from build123d import *

# Parameters (mm, degrees)
CHAMFER1_SIZE  = 0.25
FILLET1_R      = 1
SKETCH2_R      = 4
EXTRUDE1_DEPTH = 13
SKETCH3_R      = 3
EXTRUDE2_DEPTH = 8
SKETCH4_R      = 2.5
EXTRUDE3_DEPTH = 3
CHAMFER2_SIZE  = 1
CHAMFER3_SIZE2 = 0.5
CHAMFER3_SIZE  = 1
HOLEWZD1_D     = 2.5
HOLEWZD1_DEPTH = 5.5
HOLEWZD1_TIP   = 0.751075774


with BuildPart() as part:
    # Sketch1 → Revolve1 (revolve)
    with BuildSketch(Plane.XY, mode=Mode.PRIVATE) as revolve1_sk:
        Polygon((0, 0), (31, 0), (31, 12), (13.2, 12), (13.2, 10.7), (12, 10.7), (12, 12), (11, 12), (11, 6), (10, 6), (10, 2), (0, 2), align=None)
    revolve(revolve1_sk.sketch.rotate(Axis((0, 0, 0), (-1, 0, 0)), 90), axis=Axis((0, 0, 0), (-1, 0, 0)))

    # Chamfer1
    chamfer1_edges = [part.edges().sort_by_distance(p)[0] for p in [
        (0, 0, 2),
    ]]
    chamfer(chamfer1_edges, length=CHAMFER1_SIZE)

    # Fillet1
    fillet1_edges = [part.edges().sort_by_distance(p)[0] for p in [
        (31, 0, 12),
    ]]
    fillet(fillet1_edges, radius=FILLET1_R)

    # Sketch2 → Extrude1 (add)
    with BuildSketch(Plane(origin=(0, 0, 0), x_dir=(1, 0, 0), z_dir=(0, 1, 0))):
        with Locations(Location((25, 0, 0), (0, 0, 270))):
            Circle(SKETCH2_R)
    extrude(amount=-EXTRUDE1_DEPTH)

    # Sketch3 → Extrude2 (add)
    with BuildSketch(Plane.XZ.offset(13)):
        with Locations(Location((25, 0, 0), (0, 0, 90))):
            Circle(SKETCH3_R)
    extrude(amount=EXTRUDE2_DEPTH)

    # Sketch4 → Extrude3 (add)
    with BuildSketch(Plane.XZ.offset(21)):
        with Locations(Location((25, 0, 0), (0, 0, 270))):
            Circle(SKETCH4_R)
    extrude(amount=EXTRUDE3_DEPTH)

    # Chamfer2
    chamfer2_edges = [part.edges().sort_by_distance(p)[0] for p in [
        (25, -13, -4),
    ]]
    chamfer(chamfer2_edges, length=CHAMFER2_SIZE - 0.0001)  # a hair under: the kernel refuses the full size

    # Chamfer3
    chamfer3_edges = [part.edges().sort_by_distance(p)[0] for p in [
        (25, -21, -3),
    ]]
    chamfer3_side = [part.faces().sort_by_distance(p)[0] for p in [
        (25, -20.99, -3),
    ]]
    chamfer(chamfer3_edges, length=CHAMFER3_SIZE - 0.0001, length2=CHAMFER3_SIZE2 - 0.0001, reference=chamfer3_side[0])  # a hair under: the kernel refuses the full size

    # HoleWzd1
    with Locations(Plane.ZY.offset(-11)):
        with Locations((0, 9), (7.794228634, -4.5), (-7.794228634, -4.5)):
            Hole(HOLEWZD1_D / 2, depth=HOLEWZD1_DEPTH)
            with Locations((0, 0, -(HOLEWZD1_DEPTH + HOLEWZD1_TIP / 2))):  # 118° drill point
                Cone(0, HOLEWZD1_D / 2, HOLEWZD1_TIP, mode=Mode.SUBTRACT)


solid = part.part
Could you check a few things on this model? Use its own coordinates, in mm. A direction names the side the tool comes from. Round coordinates to 2 decimals unless told otherwise and drop trailing zeros. Loops run counter-clockwise (first coordinate to the right, second up) from the corner with the lowest first, then second, coordinate; pieces in that order, holes last. Notation, with made-up numbers: (-12, -8) - (21, -8) arc R18 cw to (21, 17) - close; hole circle Ø6 at (80.5, -20.75). An arc over 180 degrees is marked (long way). Write item = value, one per line.
1) Imagine slicing it at D-D (y = -18). Please give me the cut outline in (x, z), and give its area (3 significant figures).
Computed:
outline = circle Ø6 at (25, 0)
area = 28.3 mm2
2) On a 3-axis mill with a long thin cutter (end or side, diameter ignored), from which of +Z, -Z, +X, -X, +Y, -Y can I reach the whole of each face in a straight line? I mean faces 1 (the flat face through (0, 0, 0)), 2 (the cylindrical face through (12.592, 10.446, 2.32)), 3 (the cylindrical face through (10.493, -1.802, -5.723)). Say none if no direction works.
Computed:
face_1 = +Z, -Z, -X, +Y, -Y
face_2 = none
face_3 = -X
3) If we mould it in two halves opening along Z, with no side actions, what happens to faces 4 (the flat face through (12, 0, -11)), 5 (the conical face through (17.12, -4.49, 7.58)), 6 (the cylindrical face through (26.201, -11.731, 3.815))? For each: pulls with the +Z half, pulls with the -Z half, needs draft (parallel to the pull), parting line crosses it, or undercut.
Computed:
face_4 = needs draft
face_5 = undercut
face_6 = parting line crosses it
4) I'm going to push flat-ended pins straight in: P1, Ø2, axis at y = 9, z = 0, coming from the -X side; P2, Ø10, axis at x = 17.5, z = 6, coming from the +Y side; P3, Ø7, axis at y = -3.5, z = 6, coming from the -X side. Where does each tip first touch, or does it pass through?
Computed:
P1 = 16.65
P2 = 11.96
P3 = 10
5) I need wall thicknesses on line 1 along Y through (x, z) = (12.2, 0); line 2 along Y through (x, z) = (14.45, 0); line 3 along Z through (x, y) = (12.25, -4.5). Which ranges of each line are inside material? Lowest first, please. Write a range as from..to.
Computed:
line_1 = -10.7..7.75, 10.25..10.7
line_2 = -12..7.75, 10.25..12
line_3 = -9.71..-9.04, -6.54..6.54, 9.04..9.71
6) Imagine slicing it at A-A (y = 0). Please give me the cut outline in (x, z).
Computed:
outline = (0, -1.75) - (0.25, -2) - (10, -2) - (10, -6) - (11, -6) - (11, -12) - (12, -12) - (12, -10.7) - (13.2, -10.7) - (13.2, -12) - (30, -12) arc R1 ccw to (31, -11) - (31, 11) arc R1 ccw to (30, 12) - (13.2, 12) - (13.2, 10.7) - (12, 10.7) - (12, 12) - (11, 12) - (11, 6) - (10, 6) - (10, 2) - (0.25, 2) - (0, 1.75) - close
7) Imagine slicing it at C-C (x = 4.5). Please give me the cut outline in (y, z).
Computed:
outline = circle Ø4 at (0, 0)
